The model under review builds one solid part; all positions refer to its coordinate system, in mm. Face numbers are marked on the shaded views. A direction names the side the tool comes from. Round coordinates to 2 decimals unless told otherwise and drop trailing zeros. Loops run counter-clockwise (first coordinate to the right, second up) from the corner with the lowest first, then second, coordinate; pieces in that order, holes last. Notation, with made-up numbers: M 20,72.25 L 58,72.25 A19 ccw 58,96.25 Z; hole C 23,86 d7. An arc over 180 degrees is marked long. One line per question, with ' | ' between items.
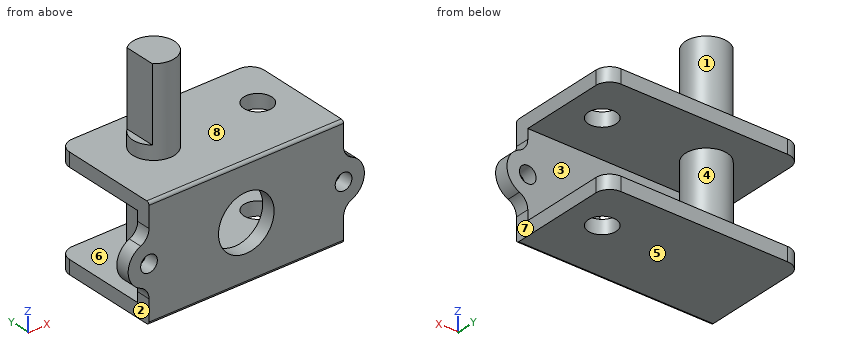
from build123d import *

# Parameters (mm, degrees)
EXTRUDE1_DEPTH      = 4
EXTRUDE2_DEPTH      = 12.357816692
EXTRUDE2_DEPTH_BACK = 12.357816692
SKETCH2_R           = 1
EXTRUDE3_DEPTH      = 12.357816692
EXTRUDE3_DEPTH_BACK = 12.357816692
SKETCH4_W           = 6
SKETCH4_H           = 8.732029078
FILLET1_R           = 0.2
FILLET2_R           = 1
EXTRUDE4_DEPTH      = 14
EXTRUDE4_DEPTH_BACK = 3
SKETCH3_R           = 1.5
EXTRUDE5_DEPTH      = 9
SKETCH6_R           = 1.5
EXTRUDE6_DEPTH      = 1
SKETCH7_R           = 0.6
EXTRUDE7_DEPTH      = 1
FILLET3_R           = 1
SKETCH8_R           = 2
EXTRUDE8_DEPTH      = 1
EXTRUDE9_START      = 6.3
SKETCH9_R           = 2.172550551
EXTRUDE9_DEPTH      = 10


with BuildPart() as part:
    # Sketch1 → Extrude1 (new, symmetric)
    with BuildSketch(Plane.XY):
        Polygon((0, 0), (-7, 0), (-7, 8), (7, 8), (7, 0), align=None)
    extrude(amount=EXTRUDE1_DEPTH, both=True)

    # Sketch2 → Extrude2 (cut, two sides: drawn at the far end of the back side and taken through both)
    with BuildSketch(Plane.XY.offset(-EXTRUDE2_DEPTH_BACK)):
        with Locations((4.5, 4.5)):
            Circle(SKETCH2_R)
    extrude(amount=EXTRUDE2_DEPTH + EXTRUDE2_DEPTH_BACK, mode=Mode.SUBTRACT)

    # Sketch4 → Extrude3 (cut, two sides: drawn at the far end of the back side and taken through both)
    with BuildSketch(Plane(origin=(0, 0, 0), x_dir=(0, 0, -1), z_dir=(1, 0, 0)).offset(-EXTRUDE3_DEPTH_BACK)):
        with Locations((0, 5.366014539)):
            Rectangle(SKETCH4_W, SKETCH4_H)
    extrude(amount=EXTRUDE3_DEPTH + EXTRUDE3_DEPTH_BACK, mode=Mode.SUBTRACT)

    # Fillet1
    fillet1_edges = [part.edges().sort_by_distance(p)[0] for p in [
        (0, 0, 4),
        (0, 0, -4),
    ]]
    fillet(fillet1_edges, radius=FILLET1_R)

    # Fillet2
    fillet2_edges = [part.edges().sort_by_distance(p)[0] for p in [
        (-7, 8, -3.5),
        (7, 8, -3.5),
        (-7, 8, 3.5),
        (7, 8, 3.5),
    ]]
    fillet(fillet2_edges, radius=FILLET2_R)

    # Sketch3 → Extrude4 (add, two sides: drawn at the far end of the back side and taken through both)
    with BuildSketch(Plane.XY.offset(-EXTRUDE4_DEPTH_BACK)):
        with Locations((-3, 4.5)):
            Circle(SKETCH3_R)
    extrude(amount=EXTRUDE4_DEPTH + EXTRUDE4_DEPTH_BACK)

    # Sketch5 → Extrude5 (cut)
    with BuildSketch(Plane.XY.offset(14)):
        Polygon((-4, 4.5), (-4, 6.060686456), (-4.95644391, 6.060686456), (-4.95644391, 2.5), (-4, 2.5), align=None)
    extrude(amount=-EXTRUDE5_DEPTH, mode=Mode.SUBTRACT)

    # Sketch6 → Extrude6 (add)
    with BuildSketch(Plane.XZ):
        with Locations((-7, 0)):
            Circle(SKETCH6_R)
        with Locations((7, 0)):
            Circle(SKETCH6_R)
    extrude(amount=-EXTRUDE6_DEPTH)

    # Sketch7 → Extrude7 (cut)
    with BuildSketch(Plane.XZ):
        with Locations((-7, 0)):
            Circle(SKETCH7_R)
        with Locations((7, 0)):
            Circle(SKETCH7_R)
    extrude(amount=-EXTRUDE7_DEPTH, mode=Mode.SUBTRACT)

    # Fillet3
    fillet3_edges = [part.edges().sort_by_distance(p)[0] for p in [
        (7, 0.5, -1.5),
        (7, 0.5, 1.5),
        (-7, 0.5, 1.5),
        (-7, 0.5, -1.5),
    ]]
    fillet(fillet3_edges, radius=FILLET3_R)

    # Sketch8 → Extrude8 (cut)
    with BuildSketch(Plane.XZ):
        Circle(SKETCH8_R)
    extrude(amount=-EXTRUDE8_DEPTH, mode=Mode.SUBTRACT)

    # Sketch9 → Extrude9 (cut)
    with BuildSketch(Plane.XY.offset(4).offset(EXTRUDE9_START)):
        with Locations((-3, 4.5)):
            Circle(SKETCH9_R)
    extrude(amount=EXTRUDE9_DEPTH, mode=Mode.SUBTRACT)


solid = part.part
1) Add section A-A on y = 2.5. State the section outline as (x, z) points.
Output values:
outline: M -7,-4 L 7,-4 L 7,-3 L -7,-3 Z; M -7,3 L 7,3 L 7,4 L -7,4 Z
2) Mouldability with a two-part tool opening along Z and no side actions: class the marked faces 5, 6, 7 and 8 as +Z half, -Z half, draft (parallel to the pull), parting line (faces both ways), or undercut.
Output values:
face 5: -Z half | face 6: undercut | face 7: draft | face 8: +Z half
3) Machinability: for the marked faces 1, 2, 3 and 4, which of the approach directions +Z, -Z, +X, -X, +Y, -Y give a long, thin tool a straight path to every point of the face, cutting with its end or side? Answer none if there is none.
Output values:
face 1: +Z | face 2: -Z, -X, +Y, -Y | face 3: +X, -X | face 4: none
4) Add section C-C on z = 0. State the section outline as (x, y) points, then the cut area to 3 significant figures.
Output values:
outline: M -8.5,0 L -7.6,0 L -7.6,1 L -8.5,1 Z; M -6.4,0 L -2,0 L -2,1 L -6.4,1 Z; C -3,4.5 d3; M 2,0 L 6.4,0 L 6.4,1 L 2,1 Z; M 7.6,0 L 8.5,0 L 8.5,1 L 7.6,1 Z | area: 17.7 mm²
5) Add section B-B on y = 4.5. State the section outline as (x, z) points.
Output values:
outline: M -7,-4 L 3.5,-4 L 3.5,-3 L -1.5,-3 L -1.5,3 L 3.5,3 L 3.5,4 L -1.5,4 L -1.5,10.3 L -4,10.3 L -4,5 L -4.5,5 L -4.5,4 L -7,4 L -7,3 L -4.5,3 L -4.5,-3 L -7,-3 Z; M 5.5,-4 L 7,-4 L 7,-3 L 5.5,-3 Z; M 5.5,3 L 7,3 L 7,4 L 5.5,4 Z
6) For line 1 (Y direction, x = 4.5, z = 3.65); line 2 (Z direction, x = 0.5, y = 7); line 3 (Z direction, x = 0, y = 0.8), list the stretches that pass through material, from the lowest coordinate up.
Output values:
line 1: y = 0 to 3.5, 5.5 to 8 | line 2: z = -4 to -3, 3 to 4 | line 3: z = -4 to -2, 2 to 4
7) Add section D-D on x = 4.5. State the section outline as (y, z) points, then the cut area to 3 significant figures.
Output values:
outline: M 0,-3.8 A0.2 ccw 0.2,-4 L 3.5,-4 L 3.5,-3 L 1,-3 L 1,3 L 3.5,3 L 3.5,4 L 0.2,4 A0.2 ccw 0,3.8 Z; M 5.5,-4 L 8,-4 L 8,-3 L 5.5,-3 Z; M 5.5,3 L 8,3 L 8,4 L 5.5,4 Z | area: 18.0 mm²
8) Insertion check: P1, Ø1, axis at y = 5, z = -0.5, coming from the -X side; P2, Ø1.4, axis at y = 3.5, z = 3, coming from the +X side; P3, Ø1, axis at y = 3.5, z = 0, coming from the +X side. Each pin has a flat end and moves straight along its axis. Give the tip position at first contact, or say it passes through.
Output values:
P1: stops at x = -4.5 | P2: stops at x = 7 | P3: stops at x = -1.59
